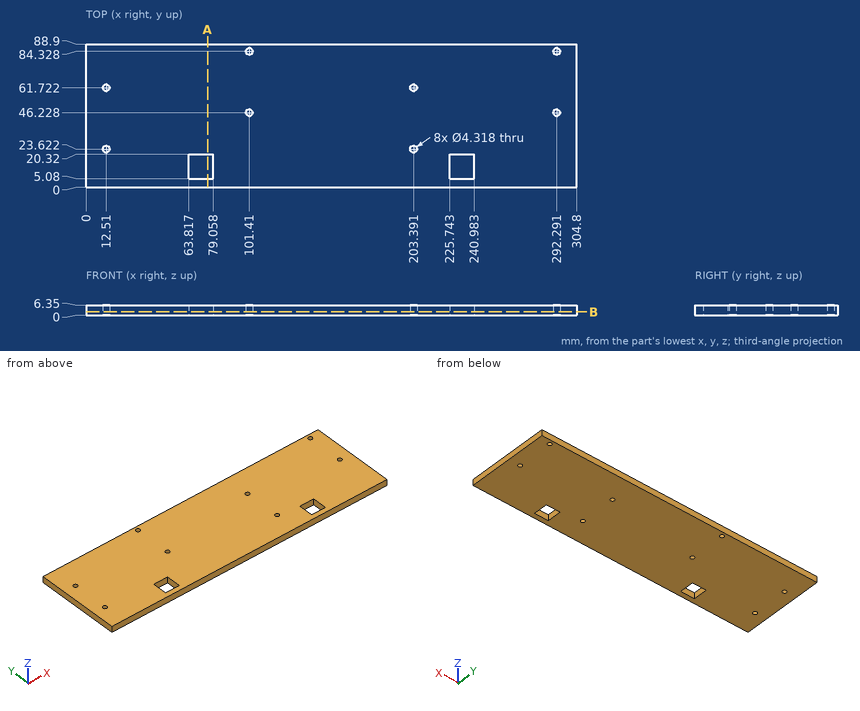
Job drawing, mm, ordinate dimensions from the low corner. One solid piece. Give positions to 0.01 mm unless a question says otherwise; leave off trailing zeros. Loops run counter-clockwise (first coordinate to the right, second up) from the corner with the lowest first, then second, coordinate; pieces in that order, holes last. Notation, with made-up numbers: M 4.25,8 L 58.25,8 A34 ccw 58.25,44 Z; hole C 74.5,25.25 d5. An arc over 180 degrees is marked long. Put each result on its own line as item: value. Start each with the question number.
1) Saw through at A-A (x = 75.5). List the corners of the cut face in (y, z), then the cut area to 3 significant figures.
2) Probe probe 1 along X at (y, z) = (20, 4); probe 2 along X at (y, z) = (45, 2) (1 decimal); probe 3 along Y at (x, z) = (14, 4) (1 decimal). List the from-to ranges inside material, lowest first.
3) Saw through at B-B (z = 2.25). State how many separate pieces and enclosed holes the cut face has, then the cut area to 3 significant figures.
4) Flat gauge pin, fed straight in: pin 1 (4 mm diameter, centred on x = 101.41, y = 84.33, fed in from +Z). Where does the tip first touch, or does it go through?
Numbers:
1. outline: M 0,0 L 5.08,0 L 5.08,6.35 L 0,6.35 Z; M 20.32,0 L 88.9,0 L 88.9,6.35 L 20.32,6.35 Z
1. area: 468 mm^2
2. probe 1: 0 to 63.82, 79.06 to 225.74, 240.98 to 304.8
2. probe 2: 0 to 99.6, 103.2 to 290.5, 294.1 to 304.8
2. probe 3: 0 to 22.1, 25.2 to 60.2, 63.3 to 88.9
3. separate pieces: 1
3. enclosed holes: 10
3. area: 26,500 mm^2
4. pin 1: through
